The model under review builds one solid part; all positions refer to its coordinate system, in mm. A direction names the side the tool comes from. Round coordinates to 2 decimals unless told otherwise and drop trailing zeros. Order: outer loops, then holes, each group sorted by start corner. A loop starts at its lowest first (then second) coordinate and runs counter-clockwise, first axis right, second up. Notation, with made-up numbers: (10.5, -14) - (38.5, -14) arc R15 cw to (38.5, 4) - close; hole circle Ø11 at (56, 75.5). An arc over 180 degrees is marked (long way). One line per question, with ' | ' between items. Start each with the question number.
Item 1: Tool access review of faces 4 (the face through (12, 0, 17)), 5 (the face through (0, -8, 5)), 6 (the face through (6.9, 16.93, 7.4)), 7 (the face through (12.5, -16.7, 17.4)): name each direction out of +Z, -Z, +X, -X, +Y, -Y from which nothing blocks a thin tool from reaching the whole face with its end or side.
Item 2: Draft analysis for pull direction Y (two halves, no side actions). For faces 1 (the face through (6.9, -16.93, 7.4)), 2 (the face through (-7.5, 0, 9)), 3 (the face through (0.12, -9.269, 10.745)), state which applies: +Y half, -Y half, draft (parallel to the pull), parting line (faces both ways), or undercut.
Item 3: Add section B-B on y = -15. State the section outline as (x, z) points.
Item 4: For L1, parallel to Y at x = 0, z = 8.25; L2, parallel to X at y = 9.5, z = 8; L3, parallel to Y at x = 1, z = 5.75, list the stretches that pass through material, from the lowest coordinate up. Write a range as [from, to].
Item 5: Add section C-C on x = 12.25. State the section outline as (y, z) points, and give its area (3 significant figures).
Item 6: Insertion check: pin 1 Ø1.8 at (x, y) = (12, -5) entering from -Z; pin 2 Ø4.5 at (y, z) = (2, 5.5) entering from +X. Each pin has a flat end and moves straight along its axis. Give the tip position at first contact, or say it passes through.
Item 7: Add section A-A on z = 3.25. State the section outline as (x, y) points, and give its area (3 significant figures).
from build123d import *

# Parameters (mm, degrees)
F0_W         = 15
F0_H         = 35
F1_DEPTH     = 17
F2_W         = 23
F2_H         = 35
F3_DEPTH     = 3
F5_D         = 3
F5_DEPTH     = 10
F5_TIP       = 0.9012909285
F6_F1_R      = 2
F6_F2_R      = 2
F6_F3_R      = 2
F6_F4_R      = 2
F6_T5_DEPTH  = 20
F6_T7_DEPTH  = 11
F6_T10_ANGLE = 90
F6_T11_DEPTH = 20
F6_T13_DEPTH = 11
F6_T16_ANGLE = 90


# Not quite as in the source:
# - a fillet or chamfer that OpenCascade refuses, or shapes differently, is made with other operations: its cross-section is extruded or revolved along the edge and cut away or added


with BuildPart() as f1:
    # F0 (on Top) → F1 (new body)
    with BuildSketch(Plane.XY):
        Rectangle(F0_W, F0_H)
    extrude(amount=F1_DEPTH)

    # F2 (on face) → F3 (join)
    with BuildSketch(Plane.XY.offset(17)):
        with Locations((4, 0)):
            Rectangle(F2_W, F2_H)
    extrude(amount=F3_DEPTH)

    # F5
    with Locations(Plane(origin=(0, 0, 0), x_dir=(1, 0, 0), z_dir=(0, 0, -1))):
        with Locations((0, 9.5), (0, -9.5)):
            Hole(F5_D / 2, depth=F5_DEPTH)
            with Locations((0, 0, -(F5_DEPTH + F5_TIP / 2))):  # 118° drill point
                Cone(0, F5_D / 2, F5_TIP, mode=Mode.SUBTRACT)

    # F6: fillet of radius 2 on 8 edges, made by hand

    # F6_f1
    f6_f1_edges = [f1.edges().sort_by_distance(p)[0] for p in [
        (-7.5, 0, 20),
    ]]
    fillet(f6_f1_edges, radius=F6_F1_R)

    # F6_f2
    f6_f2_edges = [f1.edges().sort_by_distance(p)[0] for p in [
        (7.5, 0, 17),
    ]]
    fillet(f6_f2_edges, radius=F6_F2_R)

    # F6_f3
    f6_f3_edges = [f1.edges().sort_by_distance(p)[0] for p in [
        (5, -17.5, 20),
    ]]
    fillet(f6_f3_edges, radius=F6_F3_R)

    # F6_f4
    f6_f4_edges = [f1.edges().sort_by_distance(p)[0] for p in [
        (5, 17.5, 20),
    ]]
    fillet(f6_f4_edges, radius=F6_F4_R)

    # F6_s6 → F6_t5 (cut)
    with BuildSketch(Plane.XY.offset(-5)):
        with BuildLine():
            ThreePointArc((5.5, -17.5), (6.9142135624, -16.9142135624), (7.5, -15.5))
            Line((7.5, -15.5), (7.54, -15.5))
            Line((7.54, -15.5), (7.54, -17.54))
            Line((7.54, -17.54), (5.5, -17.54))
            Line((5.5, -17.54), (5.5, -17.5))
        make_face()
    extrude(amount=F6_T5_DEPTH, mode=Mode.SUBTRACT)

    # F6_s8 → F6_t7 (cut)
    with BuildSketch(Plane.YZ.offset(9.5)):
        with BuildLine():
            ThreePointArc((-17.5, 19), (-16.9142135624, 17.5857864376), (-15.5, 17))
            Line((-15.5, 17), (-15.5, 16.96))
            Line((-15.5, 16.96), (-17.54, 16.96))
            Line((-17.54, 16.96), (-17.54, 19))
            Line((-17.54, 19), (-17.5, 19))
        make_face()
    extrude(amount=F6_T7_DEPTH, mode=Mode.SUBTRACT)

    # F6_s9 → F6_t10 (revolve, cut)
    with BuildSketch(Plane.XY.offset(15)):
        with BuildLine():
            ThreePointArc((5.5, -17.5), (6.9142135624, -16.9142135624), (7.5, -15.5))
            Line((7.5, -15.5), (7.54, -15.5))
            Line((7.54, -15.5), (7.54, -17.54))
            Line((7.54, -17.54), (5.5, -17.54))
            Line((5.5, -17.54), (5.5, -17.5))
        make_face()
    revolve(axis=Axis((9.5, -17.5, 15), (0, 1, 0)), revolution_arc=F6_T10_ANGLE, mode=Mode.SUBTRACT)

    # F6_s12 → F6_t11 (cut)
    with BuildSketch(Plane.XY.offset(-5)):
        with BuildLine():
            ThreePointArc((5.5, 17.5), (6.9142135624, 16.9142135624), (7.5, 15.5))
            Line((7.5, 15.5), (7.54, 15.5))
            Line((7.54, 15.5), (7.54, 17.54))
            Line((7.54, 17.54), (5.5, 17.54))
            Line((5.5, 17.54), (5.5, 17.5))
        make_face()
    extrude(amount=F6_T11_DEPTH, mode=Mode.SUBTRACT)

    # F6_s14 → F6_t13 (cut)
    with BuildSketch(Plane.YZ.offset(9.5)):
        with BuildLine():
            ThreePointArc((17.5, 19), (16.9142135624, 17.5857864376), (15.5, 17))
            Line((15.5, 17), (15.5, 16.96))
            Line((15.5, 16.96), (17.54, 16.96))
            Line((17.54, 16.96), (17.54, 19))
            Line((17.54, 19), (17.5, 19))
        make_face()
    extrude(amount=F6_T13_DEPTH, mode=Mode.SUBTRACT)

    # F6_s15 → F6_t16 (revolve, cut)
    with BuildSketch(Plane.XY.offset(15)):
        with BuildLine():
            ThreePointArc((5.5, 17.5), (6.9142135624, 16.9142135624), (7.5, 15.5))
            Line((7.5, 15.5), (7.54, 15.5))
            Line((7.54, 15.5), (7.54, 17.54))
            Line((7.54, 17.54), (5.5, 17.54))
            Line((5.5, 17.54), (5.5, 17.5))
        make_face()
    revolve(axis=Axis((9.5, 17.5, 15), (0, 1, 0)), revolution_arc=F6_T16_ANGLE, mode=Mode.SUBTRACT)


solid = f1.part
Determined:
1) face 4: -Z, +X, +Y, -Y | face 5: -Z | face 6: -Z, +X, +Y | face 7: -Z, +X, -Y
2) face 1: -Y half | face 2: draft | face 3: undercut
3) outline: (-7.5, 0) - (7.5, 0) - (7.5, 15) arc R2 cw to (9.5, 17) - (15.5, 17) - (15.5, 20) - (-5.5, 20) arc R2 ccw to (-7.5, 18) - close
4) L1: [-17.5, -11], [-8, 8], [11, 17.5] | L2: [-7.5, -1.5], [1.5, 7.5] | L3: [-17.5, -10.62], [-8.38, 8.38], [10.62, 17.5]
5) outline: (-17.44, 18.5) arc R2 ccw to (-15.5, 17) - (15.5, 17) arc R2 ccw to (17.44, 18.5) arc R2 ccw to (15.5, 20) - (-15.5, 20) arc R2 ccw to start | area: 102 mm2
6) pin 1: z = 17 | pin 2: x = 7.5
7) outline: (-7.5, -15.5) arc R2 ccw to (-5.5, -17.5) - (5.5, -17.5) arc R2 ccw to (7.5, -15.5) - (7.5, 15.5) arc R2 ccw to (5.5, 17.5) - (-5.5, 17.5) arc R2 ccw to (-7.5, 15.5) - close; hole circle Ø3 at (0, -9.5); hole circle Ø3 at (0, 9.5) | area: 507 mm2
